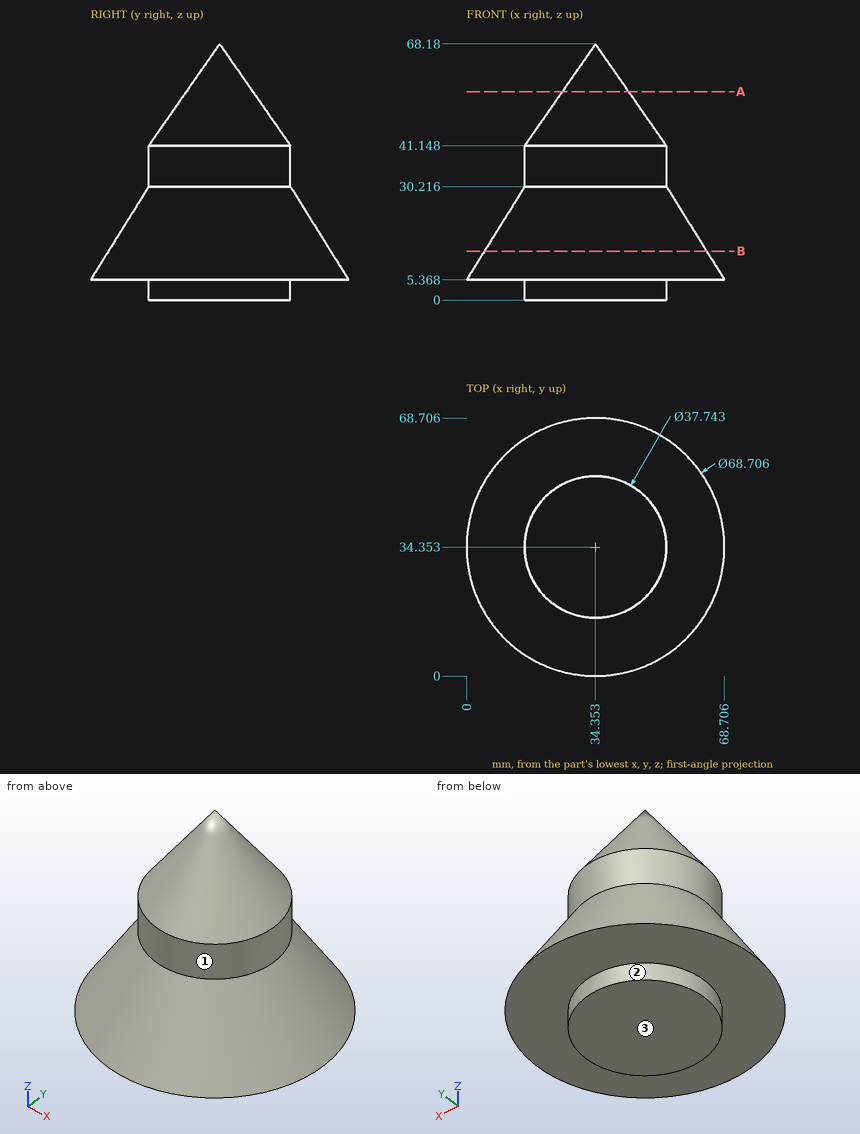
Source: three-view drawing plus pictorial views. Frame: mm from the lowest corner of the part. A direction names the side the tool comes from. Round coordinates to 2 decimals unless told otherwise and drop trailing zeros. Order: outer loops, then holes, each group sorted by start corner. A loop starts at its lowest first (then second) coordinate and runs counter-clockwise, first axis right, second up. Notation, with made-up numbers: (-21, 27) - (5, 27) arc R21 cw to (5, 50) - close; hole circle Ø2 at (48, 20). An arc over 180 degrees is marked (long way). Use a Markdown table: item, result.
1. Section A-A on z = 55.5. Return the cut outline in (x, y) (1 decimal).
Evaluation:
| item | result |
|---|---|
| outline | circle Ø17.7 at (34.4, 34.4) |
2. Material intervals for probe 1 along Z at (x, y) = (30, 49.5) (1 decimal); probe 2 along Y at (x, z) = (41, 25) (1 decimal); probe 3 along Z at (x, y) = (15.5, 7.5) (1 decimal), sorted ascending.
Evaluation:
| item | result |
|---|---|
| probe 1 | 0 to 45.6 |
| probe 2 | 13.3 to 55.5 |
| probe 3 | 5.4 to 7.8 |
3. Access query for the marked faces 1, 2 and 3. Directions: +Z, -Z, +X, -X, +Y, -Y. A direction counts if a zero-diameter tool reaches every point of the face in a straight line with its end or side. Return the directions, or none.
Evaluation:
| item | result |
|---|---|
| face 1 | +Z |
| face 2 | -Z |
| face 3 | -Z, +X, -X, +Y, -Y |
4. Section B-B on z = 13. Return the cut outline in (x, y) (1 decimal), then the cut area to 3 significant figures.
Evaluation:
| item | result |
|---|---|
| outline | circle Ø59.2 at (34.4, 34.4) |
| area | 2,750 mm^2 |
5. First-contact query: pin 1 (12 mm diameter, centred on y = 18, z = 33.5, fed in from +X); pin 2 (8 mm diameter, centred on x = 29, y = 23, fed in from +Z); pin 3 (3 mm diameter, centred on x = 56, y = 60.5, fed in from -Z). Flat tips, straight axial feed; report the tip coordinate or a pass-through.
Evaluation:
| item | result |
|---|---|
| pin 1 | x = 50.13 |
| pin 2 | z = 55.93 |
| pin 3 | z = 5.37 |
